Read the model definition and answer for the solid it produces. Units are mm, in the model's axes. Coordinates: 2 decimals unless noted, no trailing zeros. Write each loop counter-clockwise with the first axis right and the second up, starting at its lowest first coordinate (ties: lowest second). Pieces come first, ordered by that corner, then holes. Notation, with made-up numbers: (-20.5, 39) -> (7.5, 39) arc R20 cw to (7.5, 50) -> close; hole circle Ø2 at (61.5, 80). An arc over 180 degrees is marked (long way). Use CSV: the item, a comma, the result in double quotes.
from build123d import *

# Parameters (mm, degrees)
F0_W     = 57.848958
F0_H     = 84.902698
F0_R     = 3.96875
F1_DEPTH = 3.175


with BuildPart() as f1:
    # F0 (on Front) → F1 (new body)
    with BuildSketch(Plane.XZ):
        with Locations((17.556151, -32.809856)):
            Rectangle(F0_W, F0_H)
        Circle(F0_R, mode=Mode.SUBTRACT)
        with Locations((31.75, 0)):
            Circle(F0_R, mode=Mode.SUBTRACT)
    extrude(amount=F1_DEPTH)


solid = f1.part
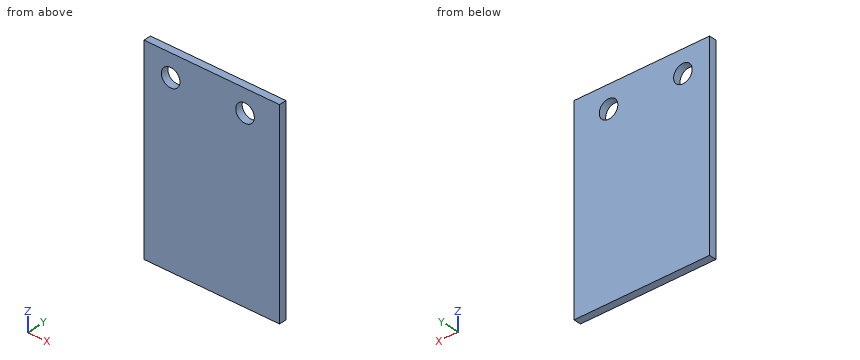
1. Find the intervals of material crossed by line 1 along Z through (x, y) = (0, -2.5); line 2 along X through (y, z) = (-1.65, -1); line 3 along Z through (x, y) = (29, -2.05), in increasing order.
Solutions:
line 1,"z = -75.26 to -3.97, 3.97 to 9.64"
line 2,"x = -11.37 to -3.84, 3.84 to 27.91, 35.59 to 46.48"
line 3,"z = -75.26 to -2.86, 2.86 to 9.64"
2. A cutting plane is placed at A-A (x = 0). Give the vertices of the cut face in (y, z) (1 decimal).
Solutions:
outline,"(-3.2, -75.3) -> (0, -75.3) -> (0, -4) -> (-3.2, -4) -> close; (-3.2, 4) -> (0, 4) -> (0, 9.6) -> (-3.2, 9.6) -> close"
3. A cutting plane is placed at B-B (y = -2.35). Give the vertices of the cut face in (x, z).
Solutions:
outline,"(-11.37, -75.26) -> (46.48, -75.26) -> (46.48, 9.64) -> (-11.37, 9.64) -> close; hole circle Ø7.94 at (0, 0); hole circle Ø7.94 at (31.75, 0)"
